from build123d import *

# Parameters (mm, degrees)
F1_DEPTH = 5
F2_R     = 0.3


with BuildPart() as f1:
    # F0 (on Front) → F1 (new body, symmetric)
    with BuildSketch(Plane.XZ):
        Polygon((0, 2.83), (0, 0), (40, 0), (40, 3.6), (20, 3.6), (20, 2.83), align=None)
    extrude(amount=F1_DEPTH, both=True)

    # F2
    f2_edges = [f1.edges().sort_by_distance(p)[0] for p in [
        (10, 5, 2.83),
        (0, 0, 2.83),
        (0, 5, 1.415),
        (0, -5, 1.415),
        (0, 0, 0),
        (20, -5, 0),
        (10, -5, 2.83),
        (20, 0, 2.83),
        (20, 5, 3.215),
        (20, -5, 3.215),
        (20, 0, 3.6),
        (30, -5, 3.6),
        (30, 5, 3.6),
        (40, 0, 3.6),
        (40, -5, 1.8),
        (40, 5, 1.8),
        (40, 0, 0),
        (20, 5, 0),
    ]]
    fillet(f2_edges, radius=F2_R)


solid = f1.part
Geometry: final body of the model. Coordinates: model frame, mm. A direction names the side the tool comes from. Give positions to 0.01 mm unless a question says otherwise; leave off trailing zeros. Write each loop counter-clockwise with the first axis right and the second up, starting at its lowest first coordinate (ties: lowest second). Pieces come first, ordered by that corner, then holes. Notation, with made-up numbers: (-13, 22) - (15, 22) arc R18 ccw to (15, 33) - close; hole circle Ø3 at (72, 39). An arc over 180 degrees is marked (long way). Return JSON: item names as keys, results as strings. Group by question number.
1) Line query: line 1 (Z direction, x = 11, y = -4.5); line 2 (Y direction, x = 38, z = 0.1); line 3 (X direction, y = -3.25, z = 2.7). Output: solid intervals per line, ascending.
2) First-contact query: P1, Ø4, axis at x = 14, y = -1, coming from the +Z side. Flat tip, straight axial feed; report the tip coordinate or a pass-through.
3) Set-up query: faces 1 (the flat face through (10, 0, 2.83)), 2 (the flat face through (40, 0, 2)). Return all of +Z, -Z, +X, -X, +Y, -Y with unobstructed straight access to the full face (end or side cutting, diameter ignored); none if empty.
4) Section A-A on x = 5.5. Return the cut outline in (y, z), plus the area to 3 significant figures.
5) Section B-B on y = 3.75. Return the cut outline in (x, z).
Filled in:
{
 "1": {"line 1": "z = 0 to 2.83", "line 2": "y = -4.92 to 4.92", "line 3": "x = 0.05 to 40"},
 "2": {"P1": "stops at z = 2.83"},
 "3": {"face 1": "+Z, -X, +Y, -Y", "face 2": "+Z, -Z, +X, +Y, -Y"},
 "4": {"outline": "(-5, 0.3) arc R0.3 ccw to (-4.7, 0) - (4.7, 0) arc R0.3 ccw to (5, 0.3) - (5, 2.53) arc R0.3 ccw to (4.7, 2.83) - (-4.7, 2.83) arc R0.3 ccw to (-5, 2.53) - close", "area": "28.2 mm^2"},
 "5": {"outline": "(0, 0.3) arc R0.3 ccw to (0.3, 0) - (39.7, 0) arc R0.3 ccw to (40, 0.3) - (40, 3.3) arc R0.3 ccw to (39.7, 3.6) - (20.3, 3.6) arc R0.3 ccw to (20, 3.3) - (20, 3.13) arc R0.3 cw to (19.7, 2.83) - (0.3, 2.83) arc R0.3 ccw to (0, 2.53) - close"}
}
